from build123d import *

# Parameters (mm, degrees)
F0_R          = 26
F0_R_2        = 11
F1_DEPTH      = 6
F1_TAPER      = 7
F2_DEPTH      = 6
F2_TAPER      = -7
F3_DEPTH      = 6
F3_DEPTH_BACK = 6


with BuildPart() as f1:
    # F0 (on Top) → F1 (new body)
    with BuildSketch(Plane.XY):
        Circle(F0_R)
        Circle(F0_R_2, mode=Mode.SUBTRACT)
        Circle(F0_R_2)
    extrude(amount=F1_DEPTH, taper=F1_TAPER)

    # F0 (on Top) → F2 (join)
    with BuildSketch(Plane.XY):
        Circle(F0_R)
        Circle(F0_R_2, mode=Mode.SUBTRACT)
        Circle(F0_R_2)
    extrude(amount=-F2_DEPTH, taper=F2_TAPER)

    # F0 (on Top) → F3 (cut, two sides)
    with BuildSketch(Plane.XY) as f3_sk:
        Circle(F0_R_2)
    extrude(amount=F3_DEPTH, mode=Mode.SUBTRACT)
    extrude(f3_sk.sketch, amount=-F3_DEPTH_BACK, mode=Mode.SUBTRACT)


solid = f1.part
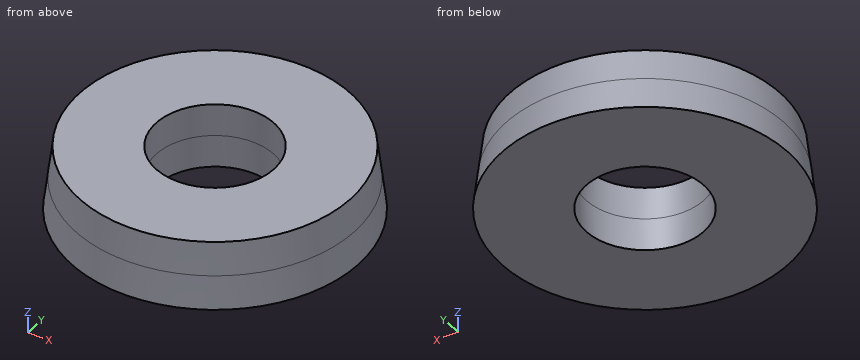
The model under review builds one solid part; all positions refer to its coordinate system, in mm. Round coordinates to 2 decimals unless told otherwise and drop trailing zeros. Write each loop counter-clockwise with the first axis right and the second up, starting at its lowest first coordinate (ties: lowest second). Pieces come first, ordered by that corner, then holes. Notation, with made-up numbers: (8.25, -20) -> (34.25, -20) arc R15 cw to (34.25, -1) -> close; hole circle Ø7 at (58, 61.5). An arc over 180 degrees is marked (long way). Answer as a JSON object with one key per item and string values.
1. To check wall thickness, follow line 1 along Y through (x, z) = (-8, 3.25); line 2 along Y through (x, z) = (0, 2.5); line 3 along X through (y, z) = (1.5, -1.25). State the ranges of each line that lie inside material, in increasing order.
Results found:
{"line 1": "y = -24.32 to -7.55, 7.55 to 24.32", "line 2": "y = -25.69 to -11, 11 to 25.69", "line 3": "x = -26.11 to -10.9, 10.9 to 26.11"}
2. We need section B-B on z = -2.5. State the section outline as (x, y) points.
Results found:
{"outline": "circle Ø52.61 at (0, 0); hole circle Ø22 at (0, 0)"}
3. Clearance check with flat-ended pins moving along their axes: pin 1 (1 mm diameter, centred on x = -7.5, z = 4.5, fed in from +Y); pin 2 (4 mm diameter, centred on x = 19.5, z = -2, fed in from -Y); pin 3 (2 mm diameter, centred on y = -7.5, z = 2.5, fed in from -X); pin 4 (13 mm diameter, centred on x = 0, y = 0, fed in from +Z). State where each tip first meets the part, or that it passes through.
Results found:
{"pin 1": "stops at y = 24.48", "pin 2": "stops at y = -19.59", "pin 3": "stops at x = -24.89", "pin 4": "passes through"}
4. We need section A-A on z = 3. State the section outline as (x, y) points.
Results found:
{"outline": "circle Ø51.26 at (0, 0); hole circle Ø22 at (0, 0)"}
